Could you check a few things on this drawing? It's one solid part, dimensions in mm from its lowest x, y, z. A direction names the side the tool comes from. Give positions to 0.01 mm unless a question says otherwise; leave off trailing zeros. Loops run counter-clockwise (first coordinate to the right, second up) from the corner with the lowest first, then second, coordinate; pieces in that order, holes last.
Q1. Suppose I cut it at C-C (x = 43.5). List the corners of the cut face in (y, z) for me, and give its area (3 significant figures).
Q2. For the marked faces 1 and 2, which set-ups out of +Z, -Z, +X, -X, +Y, -Y let a thin tool reach every point of the face, with its end or its side?
Q3. Suppose I cut it at A-A (z = 16). Count the separate pieces of the cut face and the enclosed holes in it.
Q4. I need wall thicknesses on probe 1 along X at (y, z) = (21, 2.5); probe 2 along Z at (x, y) = (37, 13). Which ranges of each line are inside material? Lowest first, please.
Q5. I'm going to push flat-ended pins straight in: P1, Ø4.5, axis at x = 46.825, y = 44.455, coming from the -Z side; P2, Ø6, axis at x = 9.525, y = 44.455, coming from the +Z side. Where does each tip first touch, or does it pass through?
Q6. Thinking about a two-plate mould opening in X: for the marked faces 3, 4 and 5, which applies, pulls with the +X half, pulls with the -X half, needs draft (parallel to the pull), parting line crosses it, or undercut?
Q7. Suppose I cut it at B-B (y = 23.5). List the corners of the cut face in (x, z) for me.
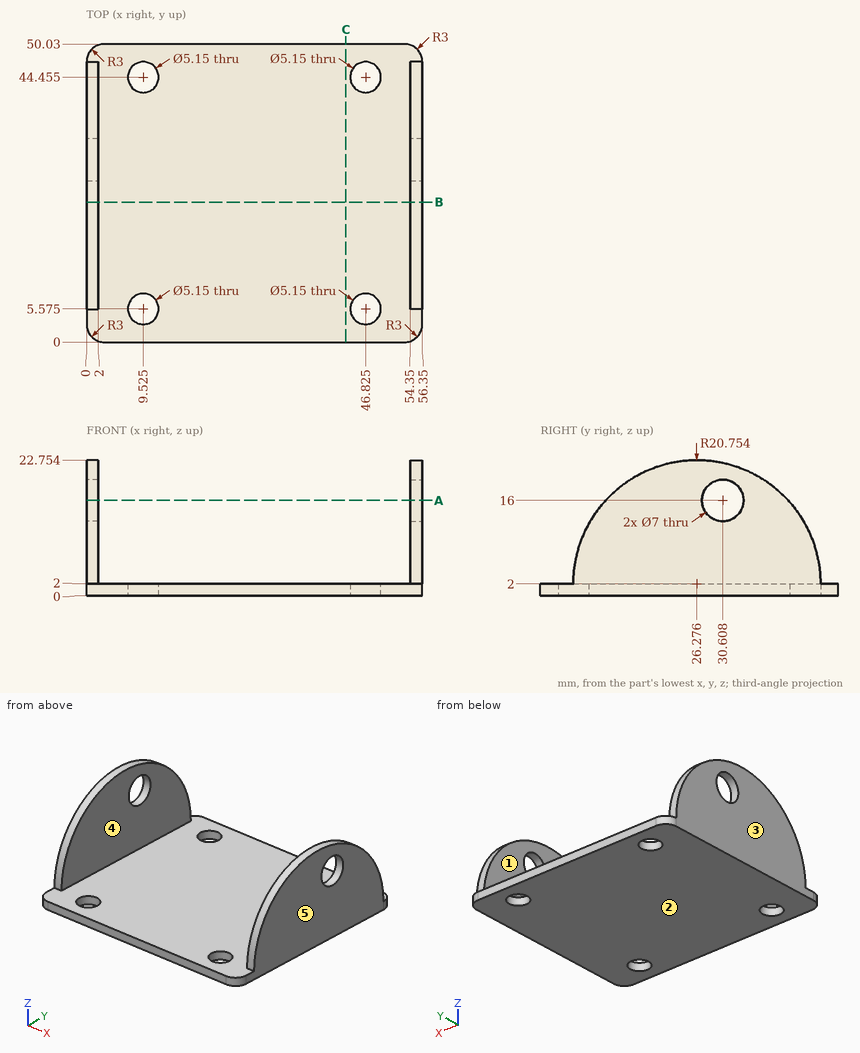
Solutions:
1. outline: (0, 0) - (50.03, 0) - (50.03, 2) - (0, 2) - close
1. area: 100 mm2
2. face 1: +Z, +Y, -Y
2. face 2: -Z, +X, -X, +Y, -Y
3. separate pieces: 4
3. enclosed holes: 0
4. probe 1: x = 0 to 2, 54.35 to 56.35
4. probe 2: z = 0 to 2
5. P1: passes through
5. P2: stops at z = 2
6. face 3: pulls with the -X half
6. face 4: undercut
6. face 5: pulls with the +X half
7. outline: (0, 0) - (56.35, 0) - (56.35, 22.57) - (54.35, 22.57) - (54.35, 2) - (2, 2) - (2, 22.57) - (0, 22.57) - close
